Read the model definition and answer for the solid it produces. Units are mm, in the model's axes. Face numbers are marked on the shaded views. A direction names the side the tool comes from. Give positions to 0.01 mm unless a question says otherwise; leave off trailing zeros. Order: outer loops, then holes, each group sorted by start corner. A loop starts at its lowest first (then second) coordinate and runs counter-clockwise, first axis right, second up.
Item 1: A cutting plane is placed at B-B (x = 2). Write down the section's boundary in (y, z), plus the area to 3 significant figures.
Item 2: Given pin 1 Ø1.3 at (x, y) = (2, -1.5) entering from -Z; pin 2 Ø1 at (y, z) = (-9, -2) entering from +X (3 decimals); pin 3 Ø4 at (x, z) = (2.5, -7) entering from -Y, each flat-ended and moving along its own axis, determine where each tip first touches the part or whether it passes through.
Item 3: A cutting plane is placed at A-A (z = 0). Write down the section's boundary in (x, y) (3 decimals), plus the area to 3 significant figures.
Item 4: A cutting plane is placed at C-C (y = 0). Write down the section's boundary in (x, z) (1 decimal).
Item 5: A cutting plane is placed at D-D (x = 9.5). Write down the section's boundary in (y, z).
Item 6: The mould has two halves that part along Z. Classify the marked faces 3, 4 and 5: +Z half, -Z half, draft (parallel to the pull), parting line (faces both ways), or undercut.
Item 7: Find the intervals of material crossed by line 1 along X through (y, z) = (6.5, 2) (3 decimals); line 2 along Y through (x, z) = (5.25, 0); line 3 along Z through (x, y) = (3, -9.25), in increasing order.
Item 8: Which of the six approach directions +Z, -Z, +X, -X, +Y, -Y give full straight-line access (tool end or side, diameter ignored) to the marked faces 1 and 2?
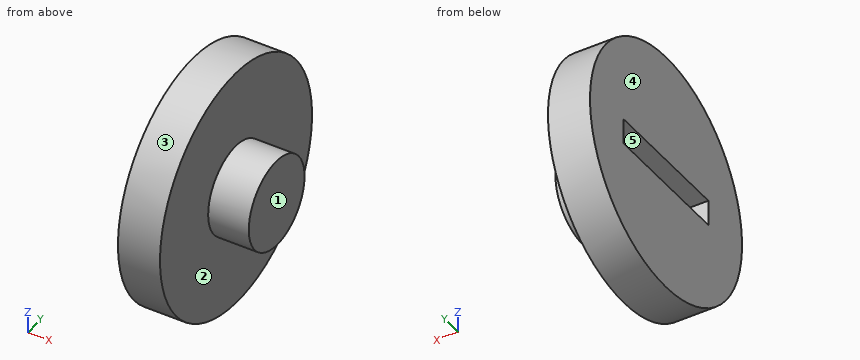
from build123d import *

# Parameters (mm, degrees)
SKETCH1_R           = 15
SKETCH1_W           = 3.175
SKETCH1_H           = 16.7
BOSS_EXTRUDE1_DEPTH = 4.175
SKETCH2_R           = 15
BOSS_EXTRUDE2_DEPTH = 1
SKETCH3_R           = 5.5
BOSS_EXTRUDE3_DEPTH = 5


with BuildPart() as part:
    # Sketch1 → Boss-Extrude1 (new body)
    with BuildSketch(Plane(origin=(0, 0, 0), x_dir=(0, 0, -1), z_dir=(1, 0, 0))):
        Circle(SKETCH1_R)
        Rectangle(SKETCH1_W, SKETCH1_H, mode=Mode.SUBTRACT)
    extrude(amount=BOSS_EXTRUDE1_DEPTH)

    # Sketch2 → Boss-Extrude2 (add)
    with BuildSketch(Plane(origin=(4.175, 0, 0), x_dir=(0, 0, -1), z_dir=(1, 0, 0))):
        Circle(SKETCH2_R)
    extrude(amount=BOSS_EXTRUDE2_DEPTH)

    # Sketch3 → Boss-Extrude3 (add)
    with BuildSketch(Plane(origin=(5.175, 0, 0), x_dir=(0, 0, -1), z_dir=(1, 0, 0))):
        Circle(SKETCH3_R)
    extrude(amount=BOSS_EXTRUDE3_DEPTH)


solid = part.part
Response values:
1. outline: circle Ø30 at (0, 0); hole (-8.35, -1.59) - (8.35, -1.59) - (8.35, 1.59) - (-8.35, 1.59) - close
1. area: 654 mm2
2. pin 1: stops at z = -14.98
2. pin 2: stops at x = 5.175
2. pin 3: stops at y = -14.14
3. outline: (0, -15) - (5.175, -15) - (5.175, -5.5) - (10.175, -5.5) - (10.175, 5.5) - (5.175, 5.5) - (5.175, 15) - (0, 15) - (0, 8.35) - (4.175, 8.35) - (4.175, -8.35) - (0, -8.35) - close
3. area: 141 mm2
4. outline: (0, -15) - (5.2, -15) - (5.2, -5.5) - (10.2, -5.5) - (10.2, 5.5) - (5.2, 5.5) - (5.2, 15) - (0, 15) - (0, 1.6) - (4.2, 1.6) - (4.2, -1.6) - (0, -1.6) - close
5. outline: circle Ø11 at (0, 0)
6. face 3: parting line
6. face 4: draft
6. face 5: undercut
7. line 1: x = 0 to 5.175
7. line 2: y = -5.5 to 5.5
7. line 3: z = -11.81 to 11.81
8. face 1: +Z, -Z, +X, +Y, -Y
8. face 2: +X
